The drawing under review shows one solid part. Ordinate dimensions are in mm from its lowest x, y, z. A direction names the side the tool comes from. Give positions to 0.01 mm unless a question says otherwise; leave off trailing zeros. Order: outer loops, then holes, each group sorted by start corner. A loop starts at its lowest first (then second) coordinate and runs counter-clockwise, first axis right, second up. Notation, with made-up numbers: (71.25, 53) - (121.25, 53) arc R16 cw to (121.25, 61) - close; hole circle Ø9 at (19, -38.5). An arc over 180 degrees is marked (long way). Use CSV: the item, a comma, the result in double quotes.
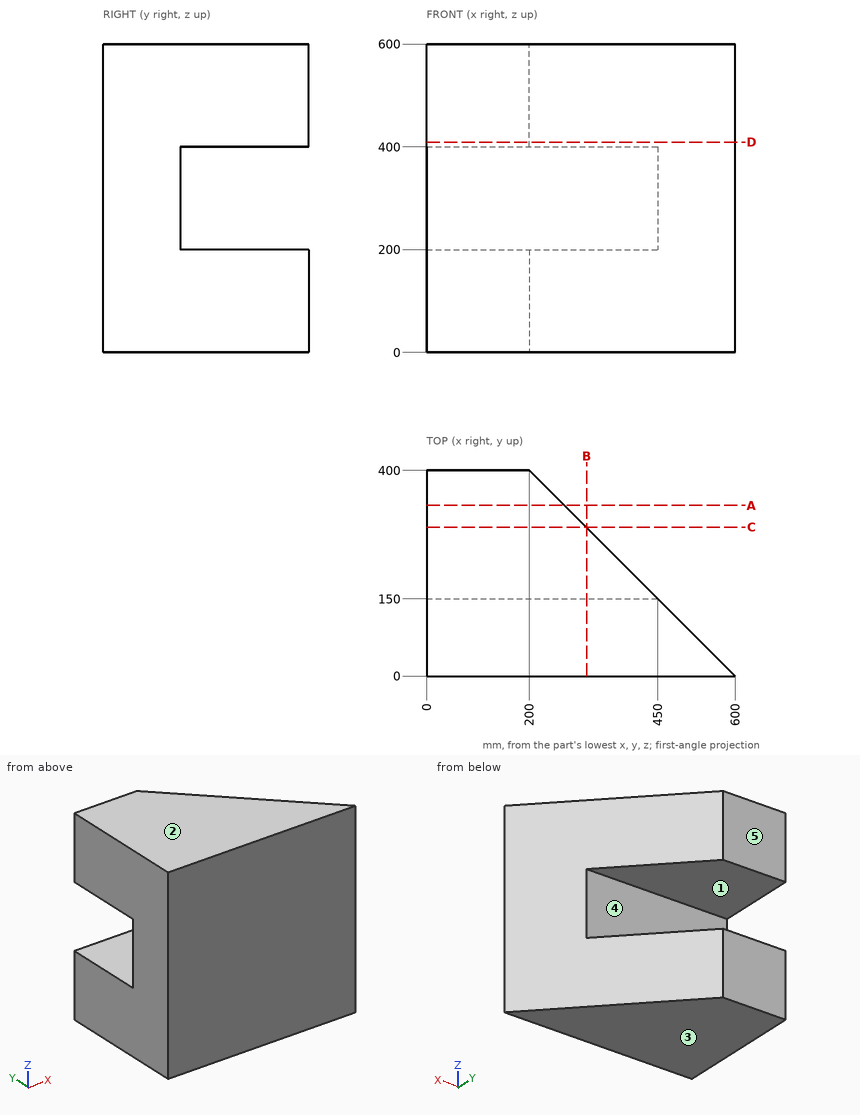
Item 1: Tool access review of the marked faces 4 and 5: name each direction out of +Z, -Z, +X, -X, +Y, -Y from which nothing blocks a thin tool from reaching the whole face with its end or side.
Results list:
face 4,"+X, -X, +Y"
face 5,"+Z, -Z, +X, -X, +Y"
Item 2: Take a section at A-A, the plane y = 332. Give the boundary of the cut face in (x, z).
Results list:
outline,"(0, 0) - (268, 0) - (268, 200) - (0, 200) - close; (0, 400) - (268, 400) - (268, 600) - (0, 600) - close"
Item 3: Take a section at C-C, the plane y = 289.5. Give the boundary of the cut face in (x, z).
Results list:
outline,"(0, 0) - (310.5, 0) - (310.5, 200) - (0, 200) - close; (0, 400) - (310.5, 400) - (310.5, 600) - (0, 600) - close"
Item 4: Wall thickness on L1, parallel to Z at x = 50.5, y = 200; L2, parallel to Y at x = 178, z = 335; L3, parallel to X at y = 106.5, z = 282: over which ranges is each line inside the solid? List them lowest first.
Results list:
L1,"z = 0 to 200, 400 to 600"
L2,"y = 0 to 150"
L3,"x = 0 to 493.5"
Item 5: Take a section at D-D, the plane z = 409. Give the boundary of the cut face in (x, y), and give its area (3 significant figures).
Results list:
outline,"(0, 0) - (600, 0) - (200, 400) - (0, 400) - close"
area,"160,000 mm2"
Item 6: Take a section at B-B, the plane x = 311.5. Give the boundary of the cut face in (y, z), and give its area (3 significant figures).
Results list:
outline,"(0, 0) - (288.5, 0) - (288.5, 200) - (150, 200) - (150, 400) - (288.5, 400) - (288.5, 600) - (0, 600) - close"
area,"145,000 mm2"
Item 7: Mouldability with a two-part tool opening along Z and no side actions: class the marked faces 1, 2 and 3 as pulls with the +Z half, pulls with the -Z half, needs draft (parallel to the pull), parting line crosses it, or undercut.
Results list:
face 1,"undercut"
face 2,"pulls with the +Z half"
face 3,"pulls with the -Z half"
Item 8: Clearance check with flat-ended pins moving along their axes: pin 1 (6 mm diameter, centred on y = 115.5, z = 393.5, fed in from +X); pin 2 (5 mm diameter, centred on x = 494, z = 144.5, fed in from +Y). State where each tip first meets the part, or that it passes through.
Results list:
pin 1,"stops at x = 487.5"
pin 2,"stops at y = 108.5"
